```python
from build123d import *

# Parameters (mm, degrees)
F1_DEPTH = 2550
F2_R     = 2
F3_R     = 1


with BuildPart() as f1:
    # F0 (on Top) → F1 (new body)
    with BuildSketch(Plane.XY):
        Polygon((20, 10), (-20, 10), (-20, -5), (-17, -5), (-17, 7), (-2, 7), (-2, -9.5), (-8.5, -9.5), (-8.5, -12.5), (0, -12.5), (8.5, -12.5), (8.5, -9.5), (2, -9.5), (2, 7), (17, 7), (17, -5), (20, -5), align=None)
    extrude(amount=F1_DEPTH)

    # F2
    f2_edges = [f1.edges().sort_by_distance(p)[0] for p in [
        (-20, 10, 1275),
        (20, 10, 1275),
    ]]
    fillet(f2_edges, radius=F2_R)

    # F3
    f3_edges = [f1.edges().sort_by_distance(p)[0] for p in [
        (-20, -5, 1275),
        (-17, -5, 1275),
        (-17, 7, 1275),
        (2, 7, 1275),
        (17, -5, 1275),
        (20, -5, 1275),
        (8.5, -12.5, 1275),
        (8.5, -9.5, 1275),
        (-8.5, -12.5, 1275),
        (-8.5, -9.5, 1275),
        (-2, 7, 1275),
        (17, 7, 1275),
        (2, -9.5, 1275),
        (-2, -9.5, 1275),
    ]]
    fillet(f3_edges, radius=F3_R)


solid = f1.part
```
Design review of the part built by this model. Coordinates are the model's own, in mm. Round coordinates to 2 decimals unless told otherwise and drop trailing zeros. Order: outer loops, then holes, each group sorted by start corner. A loop starts at its lowest first (then second) coordinate and runs counter-clockwise, first axis right, second up. Notation, with made-up numbers: M -27,87.25 L -10,87.25 A29 cw -10,109.25 Z; hole C 51.5,47 d4. An arc over 180 degrees is marked long. Put each result on its own line as item: value.
Q1. Insertion check: pin 1 Ø0.5 at (y, z) = (-11, 977.5) entering from -X; pin 2 Ø0.5 at (y, z) = (-11, 754.5) entering from +X; pin 3 Ø4 at (x, z) = (12, 1560.5) entering from -Y. Each pin has a flat end and moves straight along its axis. Give the tip position at first contact, or say it passes through.
Reported:
pin 1: x = -8.5
pin 2: x = 8.5
pin 3: y = 7
Q2. To check wall thickness, follow line 1 (X direction, y = -2, z = 546); line 2 (Y direction, x = 3.5, z = 1066); line 3 (Y direction, x = 17.5, z = 892.5). State the ranges of each line that lie inside material, in increasing order.
Reported:
line 1: -20 to -17, -2 to 2, 17 to 20
line 2: -12.5 to -9.5, 7 to 10
line 3: -4.87 to 10
Q3. Consider section A-A (y = 0.25). State the section outline as (x, z) points.
Reported:
outline: M -20,0 L -17,0 L -17,2550 L -20,2550 Z; M -2,0 L 2,0 L 2,2550 L -2,2550 Z; M 17,0 L 20,0 L 20,2550 L 17,2550 Z
